```python
from build123d import *

# Parameters (mm, degrees)
SKETCH2_R           = 4.766632538
SKETCH2_R_2         = 4.65778258
BOSS_EXTRUDE1_DEPTH = 5
SKETCH3_R           = 7.443841037
SKETCH3_R_2         = 4.766632538
BOSS_EXTRUDE2_DEPTH = 5


with BuildPart() as part:
    # Sketch2 → Boss-Extrude1 (new body)
    with BuildSketch(Plane.XY):
        with BuildLine():
            Line((-15.037844772, 149.857454221), (-25, 0))
            ThreePointArc((-25, 0), (0, -25), (25, 0))
            Line((25, 0), (1.962155228, 149.857454221))
            ThreePointArc((1.962155228, 149.857454221), (-6.537844772, 158.357454221), (-15.037844772, 149.857454221))
        make_face()
        Circle(SKETCH2_R, mode=Mode.SUBTRACT)
        with Locations((-6.537844772, 149.857454221)):
            Circle(SKETCH2_R_2, mode=Mode.SUBTRACT)
        Polygon((-19.47250371, 33.326803339), (-16.399054011, 61.179494137), (8.4679481, 61.179494137), (12.123565561, 33.326803339), align=None, mode=Mode.SUBTRACT)
        Polygon((-16.399054011, 67.186691276), (-15.037844772, 93.311013718), (5.039175994, 93.311013718), (8.4679481, 67.186691276), align=None, mode=Mode.SUBTRACT)
        Polygon((-15.037844772, 99.732600208), (-14.044403658, 124.0583194), (2.367565215, 124.0583194), (5.039175994, 99.732600208), align=None, mode=Mode.SUBTRACT)
        Polygon((-12.962496523, 141.96989308), (-14.044403658, 129.708278883), (2.367565215, 128.260163982), (0.861872424, 141.96989308), align=None, mode=Mode.SUBTRACT)
    extrude(amount=BOSS_EXTRUDE1_DEPTH)

    # Sketch3 → Boss-Extrude2 (add)
    with BuildSketch(Plane.XY.offset(5)):
        Circle(SKETCH3_R)
        Circle(SKETCH3_R_2, mode=Mode.SUBTRACT)
    extrude(amount=BOSS_EXTRUDE2_DEPTH)


solid = part.part
```
Part model, mm, in its own coordinate system. A direction names the side the tool comes from. Give positions to 0.01 mm unless a question says otherwise; leave off trailing zeros. Order: outer loops, then holes, each group sorted by start corner. A loop starts at its lowest first (then second) coordinate and runs counter-clockwise, first axis right, second up. Notation, with made-up numbers: (-22, -10) - (25, -10) arc R21 ccw to (25, 11) - close; hole circle Ø6 at (50.25, 29.25). An arc over 180 degrees is marked (long way). Use one line per item in the form item = value.
Item 1: Slice it at B-B on y = 138. Give the cut face in (x, z), and give its area (3 significant figures).
Solution:
outline = (-15.83, 0) - (-13.31, 0) - (-13.31, 5) - (-15.83, 5) - close; (1.3, 0) - (3.79, 0) - (3.79, 5) - (1.3, 5) - close
area = 25.0 mm2
Item 2: Pin check, flat tips, straight feed: pin 1 Ø1.5 at (x, z) = (0, 3) entering from -Y; pin 2 Ø15 at (x, y) = (-6.54, 149.86) entering from +Z; pin 3 Ø6 at (x, z) = (-2, 4.5) entering from +Y. Stop position of each tip, or through.
Solution:
pin_1 = -25
pin_2 = 5
pin_3 = 158.22
Item 3: Slice it at A-A on z = 2.5. Give the cut face in (x, y).
Solution:
outline = (-25, 0) arc R25 ccw to (25, 0) - (1.96, 149.86) arc R8.5 ccw to (-15.04, 149.86) - close; hole (-19.47, 33.33) - (12.12, 33.33) - (8.47, 61.18) - (-16.4, 61.18) - close; hole (-16.4, 67.19) - (8.47, 67.19) - (5.04, 93.31) - (-15.04, 93.31) - close; hole (-15.04, 99.73) - (5.04, 99.73) - (2.37, 124.06) - (-14.04, 124.06) - close; hole (-14.04, 129.71) - (2.37, 128.26) - (0.86, 141.97) - (-12.96, 141.97) - close; hole circle Ø9.32 at (-6.54, 149.86); hole circle Ø9.53 at (0, 0)
Item 4: Slice it at D-D on x = -21. Give the cut face in (y, z).
Solution:
outline = (-13.56, 0) - (60.17, 0) - (60.17, 5) - (-13.56, 5) - close
Item 5: Slice it at C-C on y = 56.5. Give the cut face in (x, z), and give its area (3 significant figures).
Solution:
outline = (-21.24, 0) - (-16.92, 0) - (-16.92, 5) - (-21.24, 5) - close; (9.08, 0) - (16.31, 0) - (16.31, 5) - (9.08, 5) - close
area = 57.8 mm2
Item 6: Two-plate mould, pull along X, no slides. Class faces 1 (the face through (-0.55, -24.994, 2.465)), 2 (the face through (2.2, -4.23, 4.93)), 3 (the face through (-19.95, 75.98, 2.46)), 4 (the face through (0, 27, 5)): released by +X, released by -X, zero draft, split by the parting line, or undercut.
Solution:
face_1 = split by the parting line
face_2 = undercut
face_3 = released by -X
face_4 = zero draft
Item 7: Which spindle directions (+Z, -Z, +X, -X, +Y, -Y) get a long thin tool onto all of the face, cutting with end or side? Do faces 5 (the face through (0, 27, 0)), 6 (the face through (-1.614, -7.267, 7.465)), 7 (the face through (-5, 99.733, 2)). Say none if no direction does.
Solution:
face_5 = -Z, +X, -X, +Y, -Y
face_6 = +Z
face_7 = +Z, -Z
Item 8: Probe probe 1 along Y at (x, z) = (-0.5, 0.75) (1 decimal); probe 2 along Y at (x, z) = (0, 2.5); probe 3 along Y at (x, z) = (0, 6.25). List the from-to ranges inside material, lowest first. Write a range as from..to.
Solution:
probe_1 = -25..-4.7, 4.7..33.3, 61.2..67.2, 93.3..99.7, 124.1..128.5, 142..155.8
probe_2 = -25..-4.77, 4.77..33.33, 61.18..67.19, 93.31..99.73, 124.06..128.47, 141.97..155.29
probe_3 = -7.44..-4.77, 4.77..7.44
